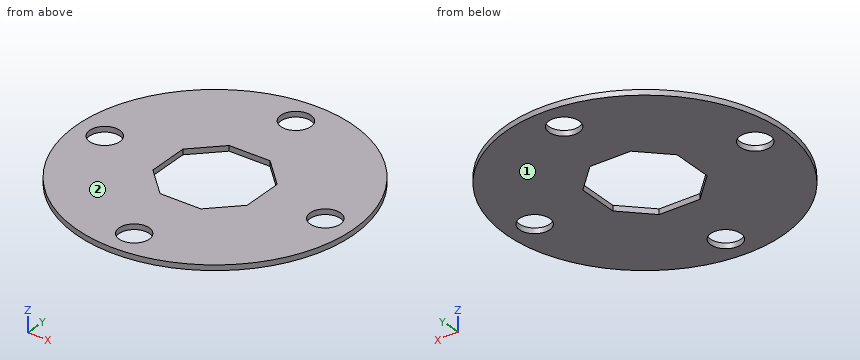
Autodesk Inventor part; units mm, degrees
ref_plane "YZ Plane" through (0, 0, 0) normal (1, 0, 0) x (0, 1, 0)
ref_plane "XZ Plane" through (0, 0, 0) normal (0, 1, 0) x (-1, 0, 0)
ref_plane "XY Plane" through (0, 0, 0) normal (0, 0, 1) x (1, 0, 0)
sketch "Sketch1" plane through (0, 0, 0) normal (0, 0, 1) x (1, 0, 0)
  circle A0 centre (0, 0) radius 78
  line L0 (26.5, 26.5) -> (-26.5, 26.5)
  line L1 (-26.5, 26.5) -> (-26.5, -26.5)
  line L2 (-26.5, -26.5) -> (26.5, -26.5)
  line L3 (26.5, -26.5) -> (26.5, 26.5)
  line L4 (26.5, 26.5) -> (-26.5, -26.5) construction
  line L5 (-26.5, 26.5) -> (26.5, -26.5) construction
  dimension "d157" = 156
  dimension "d158" = 53
  dimension "d159" = 53
extrude "Plate5" add sketch "Sketch1" along normal blind 3
sketch "Sketch7" plane through (0, 0, 0) normal (0, 0, -1) x (-1, 0, 0)
  circle A0 centre (0, 62) radius 8.5
  point P0 (0, 0)
  dimension "d160" = 17
  dimension "d161" = 62
extrude "Cut1" cut sketch "Sketch7" against normal blind 3
pattern_circular "Circular Pattern1" count 4 over 360 about axis through (0, 0, -10) along (0, 0, 1) of "Cut1"
chamfer "Corner Chamfer2" distance 15 angle 45 4 edges at (-26.5, -26.5, 1.5) (26.5, -26.5, 1.5) (-26.5, 26.5, 1.5) (26.5, 26.5, 1.5)
properties part number "PNS 1792  funnel FLANGE 1200 50-90_1600" material "Stainless Steel"
The listing builds one solid part. Answer for the finished solid, in the listing's coordinates (mm). Face numbers are marked on the shaded views. Coordinates: 2 decimals unless noted, no trailing zeros. Order: outer loops, then holes, each group sorted by start corner. A loop starts at its lowest first (then second) coordinate and runs counter-clockwise, first axis right, second up.
Q1. A cutting plane is placed at A-A, the plane x = 0. Write down the section's boundary in (y, z), and give its area (3 significant figures).
Q2. For a pull along Z with two mould halves and no side action, classify the marked faces 1 and 2 as pulls with the +Z half, pulls with the -Z half, needs draft (parallel to the pull), parting line crosses it, or undercut.
Q3. A cutting plane is placed at B-B, the plane z = 0.8. Write down the section's boundary in (x, y), and give its area (3 significant figures).
Q4. Consider line 1 (Y direction, x = 0, z = 1.05); line 2 (X direction, y = -4.5, z = 1.05); line 3 (Y direction, x = 23.5, z = 0.15). Determine where each line is inside the solid, lowest interval first.
Q5. A cutting plane is placed at C-C, the plane y = 66. Write down the section's boundary in (x, z), and give its area (3 significant figures).
Q6. Given P1, Ø0.9, axis at x = 0, z = 1.5, coming from the +Y side; P2, Ø1, axis at x = 50, z = 1.5, coming from the -Y side, each flat-ended and moving along its own axis, determine where each tip first touches the part or whether it passes through.
Q7. A cutting plane is placed at D-D, the plane x = -21. Write down the section's boundary in (y, z), and give its area (3 significant figures).
Answers follow:
1. outline: (-78, 0) - (-70.5, 0) - (-70.5, 3) - (-78, 3) - close; (-53.5, 0) - (-26.5, 0) - (-26.5, 3) - (-53.5, 3) - close; (26.5, 0) - (53.5, 0) - (53.5, 3) - (26.5, 3) - close; (70.5, 0) - (78, 0) - (78, 3) - (70.5, 3) - close
1. area: 207 mm2
2. face 1: pulls with the -Z half
2. face 2: pulls with the +Z half
3. outline: circle Ø156 at (0, 0); hole circle Ø17 at (-62, 0); hole (-26.5, -11.5) - (-11.5, -26.5) - (11.5, -26.5) - (26.5, -11.5) - (26.5, 11.5) - (11.5, 26.5) - (-11.5, 26.5) - (-26.5, 11.5) - close; hole circle Ø17 at (0, -62); hole circle Ø17 at (0, 62); hole circle Ø17 at (62, 0)
3. area: 15,800 mm2
4. line 1: y = -78 to -70.5, -53.5 to -26.5, 26.5 to 53.5, 70.5 to 78
4. line 2: x = -77.87 to -69.21, -54.79 to -26.5, 26.5 to 54.79, 69.21 to 77.87
4. line 3: y = -74.38 to -14.5, 14.5 to 74.38
5. outline: (-41.57, 0) - (-7.5, 0) - (-7.5, 3) - (-41.57, 3) - close; (7.5, 0) - (41.57, 0) - (41.57, 3) - (7.5, 3) - close
5. area: 204 mm2
6. P1: stops at y = 78
6. P2: stops at y = -60.28
7. outline: (-75.12, 0) - (-17, 0) - (-17, 3) - (-75.12, 3) - close; (17, 0) - (75.12, 0) - (75.12, 3) - (17, 3) - close
7. area: 349 mm2
